Source: three-view drawing plus pictorial views. Frame: mm from the lowest corner of the part. A direction names the side the tool comes from. Round coordinates to 2 decimals unless told otherwise and drop trailing zeros. Loops run counter-clockwise (first coordinate to the right, second up) from the corner with the lowest first, then second, coordinate; pieces in that order, holes last. Notation, with made-up numbers: (4.25, 53) -> (19.25, 53) arc R30 cw to (19.25, 89) -> close; hole circle Ø4 at (77.25, 1.5). An arc over 180 degrees is marked (long way). Put each result on its own line as item: value. Start each with the question number.
1. Cut plane C-C (z = 2.5). Return the cut outline in (x, y), then the cut area to 3 significant figures.
2. Draft query along X for the marked faces 4, 5 and 6. Return one class per face: pulls with the +X half, pulls with the -X half, needs draft (parallel to the pull), parting line crosses it, or undercut.
3. Cut plane D-D (x = 4). Return the cut outline in (y, z), then the cut area to 3 significant figures.
4. Material intervals for L1, parallel to Y at x = 54, z = 1.1; L2, parallel to X at y = 4.5, z = 5; L3, parallel to Z at x = 16, y = 13, sorted ascending.
5. Cut plane A-A (y = 8). Return the cut outline in (x, z).
6. Contact query for flat-ended pins moving along their axis: pin 1 (5 mm diameter, centred on x = 9, y = 6.5, fed in from +Z); pin 2 (2.5 mm diameter, centred on x = 27.5, y = 10, fed in from -Z); pin 3 (5 mm diameter, centred on y = 9.5, z = 8.5, fed in from +X). Output: stop coordinate, or through.
7. Set-up query: the marked faces 1, 2 and 3. Return all of +Z, -Z, +X, -X, +Y, -Y with unobstructed straight access to the full face (end or side cutting, diameter ignored); none if empty.
8. Cut plane B-B (z = 6). Return the cut outline in (x, y), then the cut area to 3 significant figures.
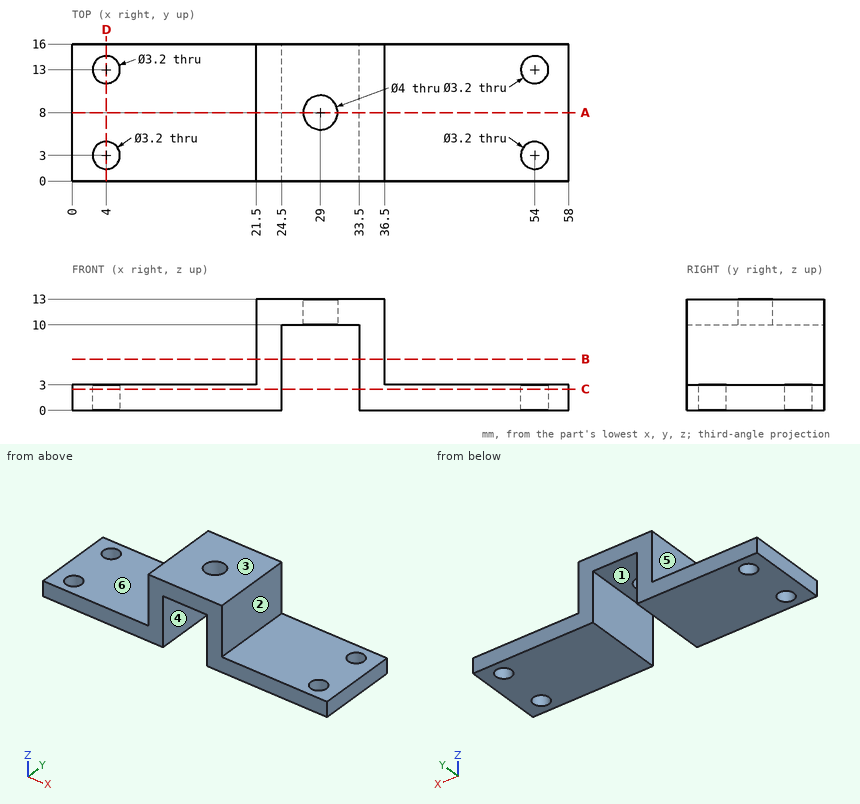
Solution:
1. outline: (0, 0) -> (24.5, 0) -> (24.5, 16) -> (0, 16) -> close; (33.5, 0) -> (58, 0) -> (58, 16) -> (33.5, 16) -> close; hole circle Ø3.2 at (4, 3); hole circle Ø3.2 at (4, 13); hole circle Ø3.2 at (54, 3); hole circle Ø3.2 at (54, 13)
1. area: 752 mm^2
2. face 4: undercut
2. face 5: pulls with the -X half
2. face 6: needs draft
3. outline: (0, 0) -> (1.4, 0) -> (1.4, 3) -> (0, 3) -> close; (4.6, 0) -> (11.4, 0) -> (11.4, 3) -> (4.6, 3) -> close; (14.6, 0) -> (16, 0) -> (16, 3) -> (14.6, 3) -> close
3. area: 28.8 mm^2
4. L1: y = 0 to 1.4, 4.6 to 11.4, 14.6 to 16
4. L2: x = 21.5 to 24.5, 33.5 to 36.5
4. L3: z = 0 to 3
5. outline: (0, 0) -> (24.5, 0) -> (24.5, 10) -> (27, 10) -> (27, 13) -> (21.5, 13) -> (21.5, 3) -> (0, 3) -> close; (31, 10) -> (33.5, 10) -> (33.5, 0) -> (58, 0) -> (58, 3) -> (36.5, 3) -> (36.5, 13) -> (31, 13) -> close
6. pin 1: stops at z = 3
6. pin 2: stops at z = 10
6. pin 3: stops at x = 36.5
7. face 1: -Z, +Y, -Y
7. face 2: +Z, +X, +Y, -Y
7. face 3: +Z, +X, -X, +Y, -Y
8. outline: (21.5, 0) -> (24.5, 0) -> (24.5, 16) -> (21.5, 16) -> close; (33.5, 0) -> (36.5, 0) -> (36.5, 16) -> (33.5, 16) -> close
8. area: 96.0 mm^2
